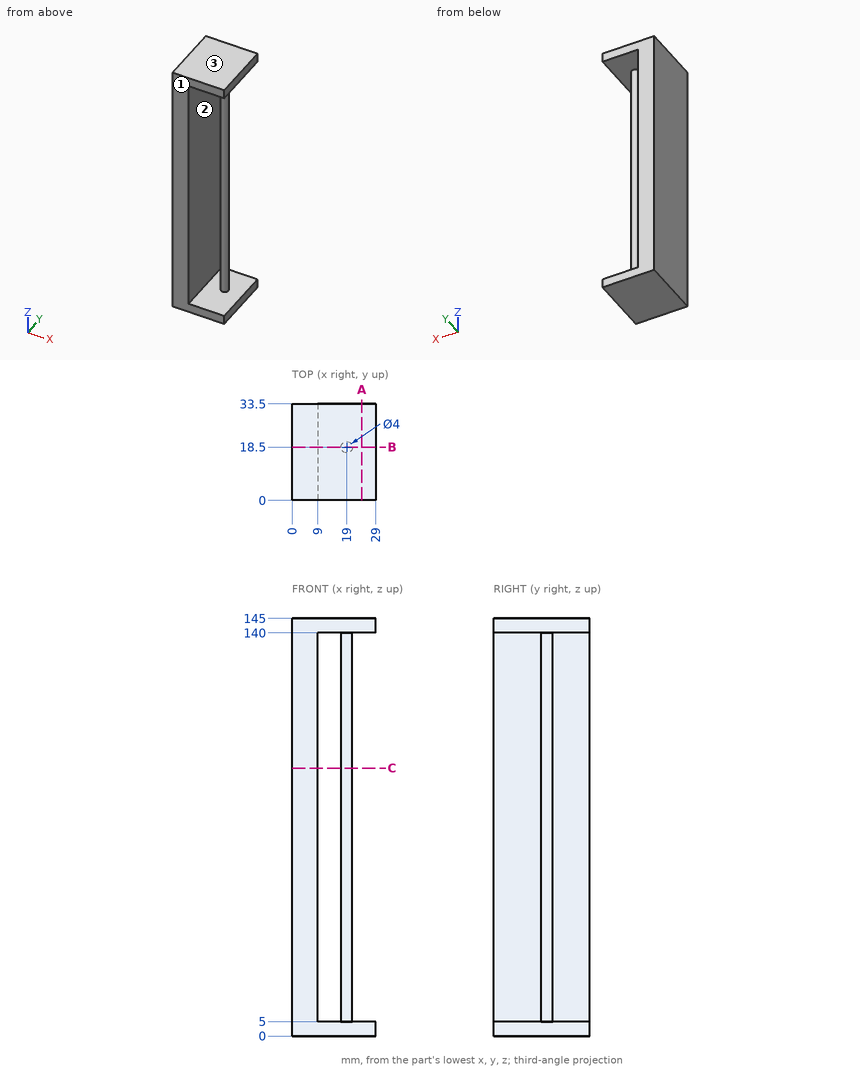
Geometry check sheet. Reference: drawing and pictorial views, mm from the part's lowest x, y, z. Give positions to 0.01 mm unless a question says otherwise; leave off trailing zeros. Write each loop counter-clockwise with the first axis right and the second up, starting at its lowest first coordinate (ties: lowest second). Pieces come first, ordered by that corner, then holes. Notation, with made-up numbers: (-10, -7.75) - (22, -7.75) arc R19 cw to (22, 15.25) - close; hole circle Ø3 at (52.25, 6). An arc over 180 degrees is marked (long way). Use a Markdown table: item, result.
Q1. Section check B-B, the plane y = 18.5. Enter the section's corners in (x, z), then the cut area to 4 significant figures.
Computed:
| item | result |
|---|---|
| outline | (0, 0) - (29, 0) - (29, 5) - (21, 5) - (21, 140) - (29, 140) - (29, 145) - (0, 145) - close; hole (9, 5) - (17, 5) - (17, 140) - (9, 140) - close |
| area | 2,045 mm² |
Q2. Section check A-A, the plane x = 24.25. Enter the section's corners in (y, z), then the cut area to 3 significant figures.
Computed:
| item | result |
|---|---|
| outline | (0, 0) - (33.5, 0) - (33.5, 5) - (0, 5) - close; (0, 140) - (33.5, 140) - (33.5, 145) - (0, 145) - close |
| area | 335 mm² |
Q3. Thickness scan on L1, parallel to Z at x = 17, y = 7; L2, parallel to X at y = 28.5, z = 52. Record the ranges inside material, lowest first. Write a range as [from, to].
Computed:
| item | result |
|---|---|
| L1 | z = [0, 5], [140, 145] |
| L2 | x = [0, 9] |
Q4. Draft check along Z on the marked faces 1, 2 and 3. Enter one of: pulls with the +Z half, pulls with the -Z half, needs draft (parallel to the pull), parting line crosses it, or undercut.
Computed:
| item | result |
|---|---|
| face 1 | needs draft |
| face 2 | undercut |
| face 3 | pulls with the +Z half |
Q5. Go/stop test with flat-tipped pins: P1, Ø4, axis at y = 19.5, z = 115.5, coming from the +X side; P2, Ø1.5, axis at y = 22.5, z = 100.5, coming from the +X side. Record where each tip stops, or that it passes through.
Computed:
| item | result |
|---|---|
| P1 | stops at x = 21 |
| P2 | stops at x = 9 |
Q6. Section check C-C, the plane z = 93. Enter the section's corners in (x, y).
Computed:
| item | result |
|---|---|
| outline | (0, 0) - (9, 0) - (9, 33.5) - (0, 33.5) - close; circle Ø4 at (19, 18.5) |
